```python
from build123d import *

# Parameters (mm, degrees)
DIKD_RTGEN_T_P_60_X_40_X_3_2_1_DEPTH = 800
IZIM3_R                              = 9
KES_EKSTR_ZYON1_DEPTH                = 50
SCALE1_SCALE                         = 0.25


with BuildPart() as part:
    # Sketch1 → Dikdörtgen tüp 60 X 40 X 3.2(1) (new body)
    with BuildSketch(Plane(origin=(0, 0, 0), x_dir=(0, 0, -1), z_dir=(1, 0, 0))):
        with BuildLine():
            Line((-13.6, -30), (13.6, -30))
            ThreePointArc((13.6, -30), (18.1254834, -28.1254834), (20, -23.6))
            Line((20, -23.6), (20, 23.6))
            ThreePointArc((20, 23.6), (18.1254834, 28.1254834), (13.6, 30))
            Line((13.6, 30), (-13.6, 30))
            ThreePointArc((-13.6, 30), (-18.1254834, 28.1254834), (-20, 23.6))
            Line((-20, 23.6), (-20, -23.6))
            ThreePointArc((-20, -23.6), (-18.1254834, -28.1254834), (-13.6, -30))
        make_face()
        with BuildLine():
            Line((-13.6, -26.8), (13.6, -26.8))
            ThreePointArc((13.6, -26.8), (15.8627417, -25.8627417), (16.8, -23.6))
            Line((16.8, -23.6), (16.8, 23.6))
            ThreePointArc((16.8, 23.6), (15.8627417, 25.8627417), (13.6, 26.8))
            Line((13.6, 26.8), (-13.6, 26.8))
            ThreePointArc((-13.6, 26.8), (-15.8627417, 25.8627417), (-16.8, 23.6))
            Line((-16.8, 23.6), (-16.8, -23.6))
            ThreePointArc((-16.8, -23.6), (-15.8627417, -25.8627417), (-13.6, -26.8))
        make_face(mode=Mode.SUBTRACT)
    extrude(amount=DIKD_RTGEN_T_P_60_X_40_X_3_2_1_DEPTH)

    # Çizim3 → Kes-Ekstrüzyon1 (cut, symmetric)
    with BuildSketch(Plane(origin=(0, 0, 0), x_dir=(1, 0, 0), z_dir=(0, 1, 0))):
        with Locations(Location((400, 0, 0), (0, 0, 270))):
            Circle(IZIM3_R)
    extrude(amount=KES_EKSTR_ZYON1_DEPTH, both=True, mode=Mode.SUBTRACT)


with BuildPart() as part_1:
    # Scale1: scaled about (0, 0, 0)
    add(part.part.scale(SCALE1_SCALE))


solid = part_1.part
```
The listing builds one solid part. Answer for the finished solid, in the listing's coordinates (mm). A direction names the side the tool comes from. Round coordinates to 2 decimals unless told otherwise and drop trailing zeros. Order: outer loops, then holes, each group sorted by start corner. A loop starts at its lowest first (then second) coordinate and runs counter-clockwise, first axis right, second up. Notation, with made-up numbers: (18, 77) - (76, 77) arc R10 ccw to (76, 88) - close; hole circle Ø1 at (71.5, 60). An arc over 180 degrees is marked (long way). Put each result on its own line as item: value. Start each with the question number.
(1) Given P1, Ø4, axis at x = 100, z = 0, coming from the -Y side, flat-ended and moving along its own axis, determine where the tip first touches the part or whether it passes through.
(2) Find section B-B (x = 100). Give the vertices of the cut face in (y, z).
(3) For faces 1 (the flat face through (98.6, -6.7, -2.2)), 2 (the flat face through (0, 1.1, 4.5)), determine the directions among +Z, -Z, +X, -X, +Y, -Y from which every point of the face is accessible in a straight line to the end or side of a thin tool.
(4) Determine the mould class of faces 3 (the flat face through (99, 0, 5)), 4 (the flat face through (98.6, 7.5, 2.2)), 5 (the flat face through (99, 0, -4.2)) for opening direction Y: released by +Y, released by -Y, zero draft, split by the parting line, or undercut.
(5) Find section C-C (z = 0). Give the vertices of the cut face in (x, y), plus the area to 3 significant figures.
(6) Find section A-A (y = 4.25). Give the vertices of the cut face in (x, z).
(7) Straight lines are drawn through the part: probe 1 along X at (y, z) = (6.9, 0); probe 2 along Z at (x, y) = (16, 4); probe 3 along Y at (x, z) = (176, -3). For each, find the intervals that lie inside material, in ascending order. Write a range as from..to.
Reply:
1. P1: through
2. outline: (-7.5, -3.4) arc R1.6 ccw to (-5.9, -5) - (5.9, -5) arc R1.6 ccw to (7.5, -3.4) - (7.5, -2.25) - (6.7, -2.25) - (6.7, -3.4) arc R0.8 cw to (5.9, -4.2) - (-5.9, -4.2) arc R0.8 cw to (-6.7, -3.4) - (-6.7, -2.25) - (-7.5, -2.25) - close; (-7.5, 2.25) - (-6.7, 2.25) - (-6.7, 3.4) arc R0.8 cw to (-5.9, 4.2) - (5.9, 4.2) arc R0.8 cw to (6.7, 3.4) - (6.7, 2.25) - (7.5, 2.25) - (7.5, 3.4) arc R1.6 ccw to (5.9, 5) - (-5.9, 5) arc R1.6 ccw to (-7.5, 3.4) - close
3. face 1: +X, -X
3. face 2: +Z, -Z, -X, +Y, -Y
4. face 3: zero draft
4. face 4: released by +Y
4. face 5: undercut
5. outline: (0, -7.5) - (97.75, -7.5) - (97.75, -6.7) - (0, -6.7) - close; (0, 6.7) - (97.75, 6.7) - (97.75, 7.5) - (0, 7.5) - close; (102.25, -7.5) - (200, -7.5) - (200, -6.7) - (102.25, -6.7) - close; (102.25, 6.7) - (200, 6.7) - (200, 7.5) - (102.25, 7.5) - close
5. area: 313 mm^2
6. outline: (0, -5) - (200, -5) - (200, -4.2) - (0, -4.2) - close; (0, 4.2) - (200, 4.2) - (200, 5) - (0, 5) - close
7. probe 1: 0..97.75, 102.25..200
7. probe 2: -5..-4.2, 4.2..5
7. probe 3: -7.5..-6.7, 6.7..7.5
